Drawing for the job (mm, zero at the part's lowest x, y, z). A direction names the side the tool comes from. Coordinates: 2 decimals unless noted, no trailing zeros. Write each loop counter-clockwise with the first axis right and the second up, starting at its lowest first coordinate (ties: lowest second). Pieces come first, ordered by that corner, then holes. Notation, with made-up numbers: M 52,-21 L 104,-21 A6 ccw 104,-14 Z; hole C 15.5,64 d4. An arc over 180 degrees is marked long. Put each result on its own line as item: value. Start each with the question number.
Q1. Pull direction Z, two halves, no side cores. Call the marked faces 3, 4, 5 and 6: pulls with the +Z half, pulls with the -Z half, needs draft (parallel to the pull), parting line crosses it, or undercut.
Q2. Drop flat-ended pins along their axis: pin 1 (4 mm diameter, centred on y = 10.5, z = 22.5, fed in from +X); pin 2 (1.5 mm diameter, centred on y = 8.5, z = 30, fed in from +X); pin 3 (12 mm diameter, centred on x = 6.5, z = 27, fed in from -Y); pin 4 (1.5 mm diameter, centred on y = 2.5, z = 21, fed in from -X). Give the stop position or say it passes through.
Q3. Cut at B-B (z = 26). Write the cut outline in (x, y), then the cut area to 3 significant figures.
Q4. Cut at A-A (x = 26). Write the cut outline in (y, z).
Q5. Which spindle directions (+Z, -Z, +X, -X, +Y, -Y) get a long thin tool onto all of the face, cutting with end or side? Do the marked faces 1 and 2. Say none if no direction does.
Q6. Cut at C-C (y = 4). Write the cut outline in (x, z).
Q7. Drill centre lines: line 1 along X through (y, z) = (9, 26); line 2 along Y through (x, z) = (27, 45.5). Where is each one in solid material? Low to high.
Q8. Cut at D-D (x = 36). Write the cut outline in (y, z), then the cut area to 3 significant figures.
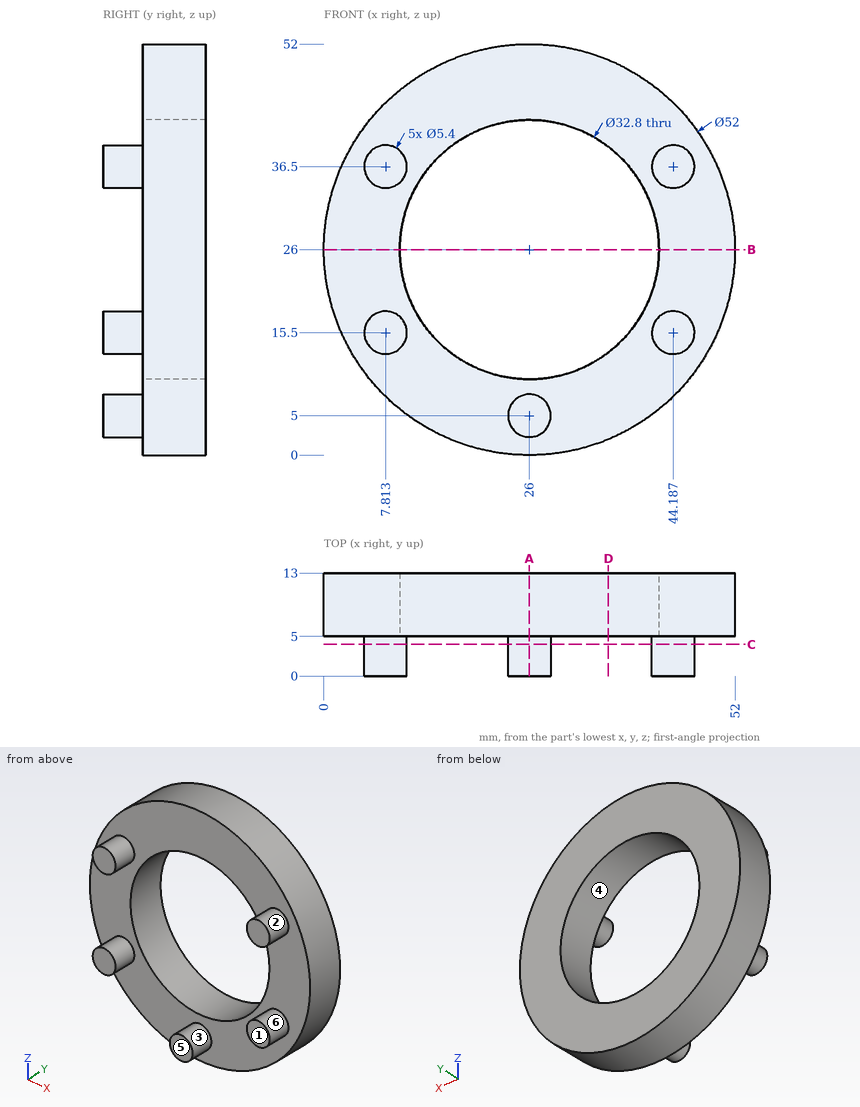
Computed values:
1. face 3: parting line crosses it
1. face 4: undercut
1. face 5: needs draft
1. face 6: undercut
2. pin 1: x = 51.96
2. pin 2: x = 51.8
2. pin 3: y = 5
2. pin 4: through
3. outline: M 0,5 L 9.6,5 L 9.6,13 L 0,13 Z; M 42.4,5 L 52,5 L 52,13 L 42.4,13 Z
3. area: 154 mm2
4. outline: M 0,2.3 L 5,2.3 L 5,0 L 13,0 L 13,9.6 L 5,9.6 L 5,7.7 L 0,7.7 Z; M 5,42.4 L 13,42.4 L 13,52 L 5,52 Z
5. face 1: +Z, -Z, +X, -X, -Y
5. face 2: -Y
6. outline: C 7.81,15.5 d5.4; C 7.81,36.5 d5.4; C 26,5 d5.4; C 44.19,15.5 d5.4; C 44.19,36.5 d5.4
7. line 1: 0 to 9.6, 42.4 to 52
7. line 2: 5 to 13
8. outline: M 5,2 L 13,2 L 13,13 L 5,13 Z; M 5,39 L 13,39 L 13,50 L 5,50 Z
8. area: 176 mm2
